Here's the drawing with two shaded views (mm, measured from the low corner). I have some questions. Coordinates: 2 decimals unless noted, no trailing zeros. Loops run counter-clockwise (first coordinate to the right, second up) from the corner with the lowest first, then second, coordinate; pieces in that order, holes last. Notation, with made-up numbers: (-12.5, 47) -> (25.5, 47) arc R21 cw to (25.5, 67) -> close; hole circle Ø5 at (48, 8). An arc over 180 degrees is marked (long way). Answer as a JSON object with one key per item and string values. Group by question number.
1) I want a section at C-C (z = 971). Write out the boundary of the cut face in (x, y).
2) I need wall thicknesses on probe 1 along X at (y, z) = (290, 444); probe 2 along Y at (x, z) = (233.5, 307); probe 3 along X at (y, z) = (60.5, 259.5). Which ranges of each line are inside material? Lowest first, please. Write a range as [from, to].
3) I'm going to push flat-ended pins straight in: pin 1 (2 mm diameter, centred on x = 249, z = 509.5, fed in from +Y); pin 2 (4 mm diameter, centred on x = 144.5, z = 131, fed in from -Y); pin 3 (2 mm diameter, centred on y = 80, z = 534.5, fed in from -X). Where does each tip first touch, or does it pass through?
4) If we mould it in two halves opening along X, with no side actions, what happens to the marked faces 1 and 2? For each: +X half, -X half, draft (parallel to the pull), parting line (faces both ways), or undercut.
5) I want a section at A-A (x = 290). Write out the boundary of the cut face in (y, z).
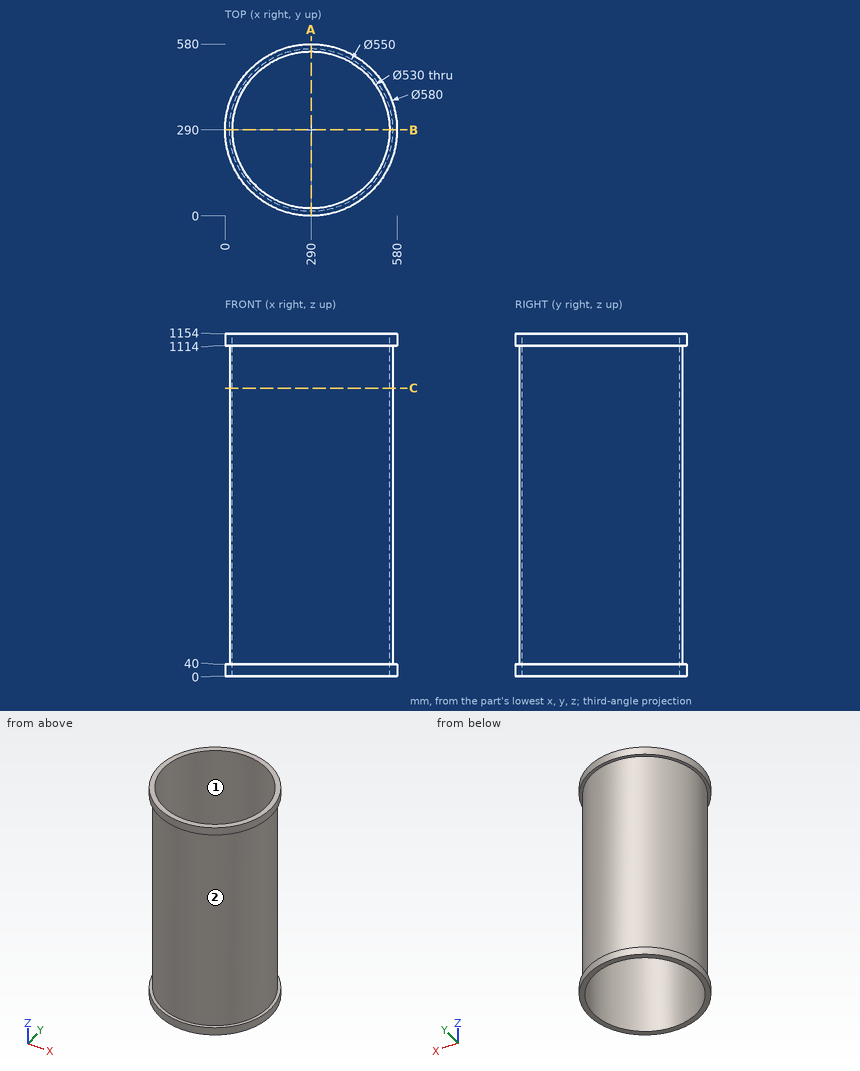
Determined:
{
 "1": {"outline": "circle Ø550 at (290, 290); hole circle Ø530 at (290, 290)"},
 "2": {"probe 1": "[15, 25], [555, 565]", "probe 2": "[20.87, 31.09], [548.91, 559.13]", "probe 3": "[138.49, 157.51], [422.49, 441.51]"},
 "3": {"pin 1": "y = 562.08", "pin 2": "y = 55.41", "pin 3": "x = 111.27"},
 "4": {"face 1": "undercut", "face 2": "parting line"},
 "5": {"outline": "(0, 0) -> (25, 0) -> (25, 1154) -> (0, 1154) -> (0, 1114) -> (15, 1114) -> (15, 40) -> (0, 40) -> close; (555, 0) -> (580, 0) -> (580, 40) -> (565, 40) -> (565, 1114) -> (580, 1114) -> (580, 1154) -> (555, 1154) -> close"}
}
